Design review of the part shown in the three views and the two pictorial views. Dimensions are in mm from the part's minimum x, y and z. Round coordinates to 2 decimals unless told otherwise and drop trailing zeros. Loops run counter-clockwise (first coordinate to the right, second up) from the corner with the lowest first, then second, coordinate; pieces in that order, holes last. Notation, with made-up numbers: (2.5, 6) -> (57.5, 6) arc R17 cw to (57.5, 29) -> close; hole circle Ø8 at (32.5, -32). An arc over 180 degrees is marked (long way). Use CSV: the item, a comma, the result in double quotes. Start each with the question number.
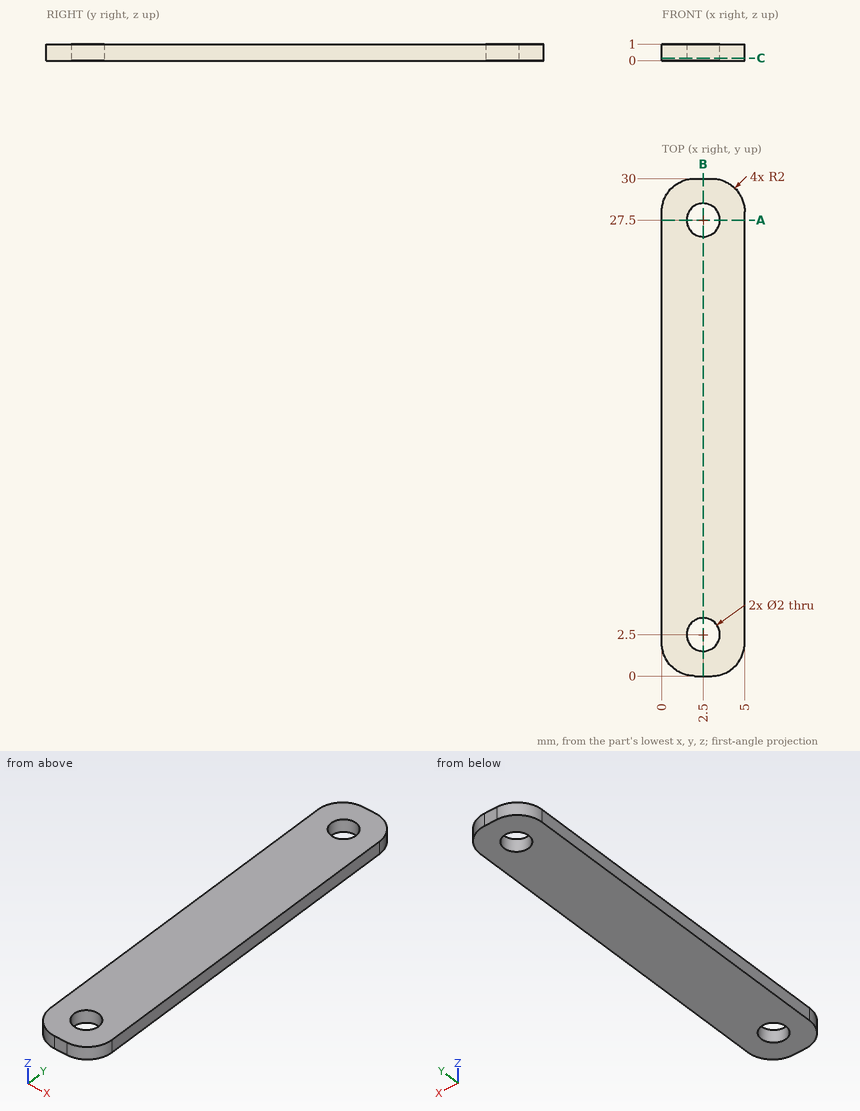
1. For line 1 along Y through (x, z) = (2.5, 0.6); line 2 along Y through (x, z) = (2.9, 0.25); line 3 along Y through (x, z) = (1.45, 0.2), list the stretches that pass through material, from the lowest coordinate up. Write a range as from..to.
2. Take a section at C-C, the plane z = 0.15. Give the boundary of the cut face in (x, y), then the cut area to 3 significant figures.
3. Take a section at B-B, the plane x = 2.5. Give the boundary of the cut face in (y, z).
4. Take a section at A-A, the plane y = 27.5. Give the boundary of the cut face in (x, z).
Results:
1,line 1,"0..1.5, 3.5..26.5, 28.5..30"
1,line 2,"0..1.58, 3.42..26.58, 28.42..30"
1,line 3,"0.08..29.92"
2,outline,"(0, 2) arc R2 ccw to (2, 0) -> (3, 0) arc R2 ccw to (5, 2) -> (5, 28) arc R2 ccw to (3, 30) -> (2, 30) arc R2 ccw to (0, 28) -> close; hole circle Ø2 at (2.5, 2.5); hole circle Ø2 at (2.5, 27.5)"
2,area,"140 mm²"
3,outline,"(0, 0) -> (1.5, 0) -> (1.5, 1) -> (0, 1) -> close; (3.5, 0) -> (26.5, 0) -> (26.5, 1) -> (3.5, 1) -> close; (28.5, 0) -> (30, 0) -> (30, 1) -> (28.5, 1) -> close"
4,outline,"(0, 0) -> (1.5, 0) -> (1.5, 1) -> (0, 1) -> close; (3.5, 0) -> (5, 0) -> (5, 1) -> (3.5, 1) -> close"
